Work out the finished part from the listing and answer in its coordinate system (mm). A direction names the side the tool comes from. Coordinates: 2 decimals unless noted, no trailing zeros. Order: outer loops, then holes, each group sorted by start corner. A loop starts at its lowest first (then second) coordinate and runs counter-clockwise, first axis right, second up. Notation, with made-up numbers: M -25.75,37 L -8.75,37 A7 cw -8.75,41 Z; hole C 80,13.25 d9. An arc over 180 degrees is marked long. Write item = value, one per line. Start each with the question number.
Q1. Determine the mould class of faces 1 (the flat face through (0, 12, 0)), 2 (the cylindrical face through (-23.78, 1.52, 9.17)), 3 (the flat face through (-16, 0, 0)) for opening direction X: released by +X, released by -X, zero draft, split by the parting line, or undercut.
Q2. Find section A-A on x = -25. Give the vertices of the cut face in (y, z).
Q3. A tool of negligible diameter and unlimited length cuts with its end or side. For faces 4 (the cylindrical face through (-12.35, 1.52, 9.06)), 5 (the flat face through (-18, 3, 0)), from which of +Z, -Z, +X, -X, +Y, -Y can it reach the whole face along a straight path? Write none if from no direction.
Q4. Find section C-C on y = 16.5. Give the vertices of the cut face in (x, z).
Q5. Find section B-B on z = -1. Give the vertices of the cut face in (x, y).
Q6. Straight lines are drawn through the part: line 1 along Y through (x, z) = (-15, 5.25); line 2 along X through (y, z) = (12, -6.75); line 3 along X through (y, z) = (2.5, 7.25). For each, find the intervals that lie inside material, in ascending order.
Q7. Find section D-D on x = -17.5. Give the vertices of the cut face in (y, z).
Q8. Each of these flat-tipped pins is pushed along its axis until it touches: P1, Ø6, axis at x = -27.5, z = -8.5, coming from the +Y side; P2, Ø1, axis at y = 10, z = 5, coming from the -X side; P3, Ø5, axis at y = 19.5, z = 0.29, coming from the +X side. Where does it stop, or does it pass through?
```python
from build123d import *

# Parameters (mm, degrees)
BOSS_EXTRUDE1_OUTLINE_W = 3
BOSS_EXTRUDE1_OUTLINE_H = 26.4
BOSS_EXTRUDE1_DEPTH     = 32.7
SKETCH2_W               = 26.4
SKETCH2_H               = 3
BOSS_EXTRUDE2_DEPTH     = 29.8
SKETCH3_R               = 2
CUT_EXTRUDE1_DEPTH      = 3
CUT_EXTRUDE3_DEPTH      = 12
SKETCH6_R               = 4
CUT_EXTRUDE4_DEPTH      = 12


# Read off the part's stored shape, not the designer's step: Boss-Extrude1
with BuildPart() as part:
    # Boss-Extrude1 outline → Boss-Extrude1 (new body)
    with BuildSketch(Plane(origin=(0, 0, 0), x_dir=(1, 0, 0), z_dir=(0, 1, 0))):
        with Locations((-1.5, -0.285443038)):
            Rectangle(BOSS_EXTRUDE1_OUTLINE_W, BOSS_EXTRUDE1_OUTLINE_H)
    extrude(amount=BOSS_EXTRUDE1_DEPTH)

    # Sketch2 → Boss-Extrude2 (add)
    with BuildSketch(Plane.ZY.offset(3)):
        with Locations((0.285443038, 1.5)):
            Rectangle(SKETCH2_W, SKETCH2_H)
    extrude(amount=BOSS_EXTRUDE2_DEPTH)

    # Sketch3 → Cut-Extrude1 (cut)
    with BuildSketch(Plane(origin=(0, 3, 0), x_dir=(1, 0, 0), z_dir=(0, 1, 0))):
        with Locations(Location((-25, 7.914556962, 0), (0, 0, 270))):
            Circle(SKETCH3_R)
        with Locations(Location((-11, 7.914556962, 0), (0, 0, 270))):
            Circle(SKETCH3_R)
        with Locations(Location((-11, -7.585443038, 0), (0, 0, 90))):
            Circle(SKETCH3_R)
        with Locations(Location((-25, -7.585443038, 0), (0, 0, 90))):
            Circle(SKETCH3_R)
    extrude(amount=-CUT_EXTRUDE1_DEPTH, mode=Mode.SUBTRACT)

    # Sketch5 → Cut-Extrude3 (cut)
    with BuildSketch(Plane.ZY.offset(3)):
        with BuildLine():
            Line((0.285443053, 32.7), (-12.914556962, 32.7))
            Line((-12.914556962, 32.7), (-12.914556962, 19.5))
            ThreePointArc((-12.914556962, 19.5), (-9.048366468, 28.833809517), (0.285443053, 32.7))
        make_face()
        with BuildLine():
            Line((13.485443038, 32.7), (0.285443053, 32.7))
            ThreePointArc((0.285443053, 32.7), (9.619252555, 28.833809506), (13.485443038, 19.5))
            Line((13.485443038, 19.5), (13.485443038, 32.7))
        make_face()
    extrude(amount=-CUT_EXTRUDE3_DEPTH, mode=Mode.SUBTRACT)

    # Sketch6 → Cut-Extrude4 (cut)
    with BuildSketch(Plane.ZY.offset(3)):
        with Locations((0.285443038, 19.5)):
            Circle(SKETCH6_R)
    extrude(amount=-CUT_EXTRUDE4_DEPTH, mode=Mode.SUBTRACT)


solid = part.part
```
Findings below:
q1.face_1 = released by +X
q1.face_2 = undercut
q1.face_3 = zero draft
q2.outline = M 0,-12.91 L 3,-12.91 L 3,-9.91 L 0,-9.91 Z; M 0,-5.91 L 3,-5.91 L 3,5.59 L 0,5.59 Z; M 0,9.59 L 3,9.59 L 3,13.49 L 0,13.49 Z
q3.face_4 = +Y, -Y
q3.face_5 = +Z, -Z, -X, +Y
q4.outline = M -3,-12.91 L 0,-12.91 L 0,-2.36 L -3,-2.36 Z; M -3,2.93 L 0,2.93 L 0,13.49 L -3,13.49 Z
q5.outline = M -32.8,0 L 0,0 L 0,15.71 L -3,15.71 L -3,3 L -32.8,3 Z; M -3,23.29 L 0,23.29 L 0,32.64 L -3,32.64 Z
q6.line_1 = 0 to 3
q6.line_2 = -3 to 0
q6.line_3 = -32.8 to -26.97, -23.03 to -12.97, -9.03 to 0
q7.outline = M 0,-12.91 L 3,-12.91 L 3,13.49 L 0,13.49 Z
q8.P1 = 3
q8.P2 = -3
q8.P3 = through
